Source: three-view drawing plus pictorial views. Frame: mm from the lowest corner of the part. A direction names the side the tool comes from. Coordinates: 2 decimals unless noted, no trailing zeros. Write each loop counter-clockwise with the first axis right and the second up, starting at its lowest first coordinate (ties: lowest second). Pieces come first, ordered by that corner, then holes. Notation, with made-up numbers: (70, 55) - (124, 55) arc R13 ccw to (124, 74) - close; hole circle Ø7 at (-34, 56). An arc over 180 degrees is marked (long way). Put each result on its own line as item: value.
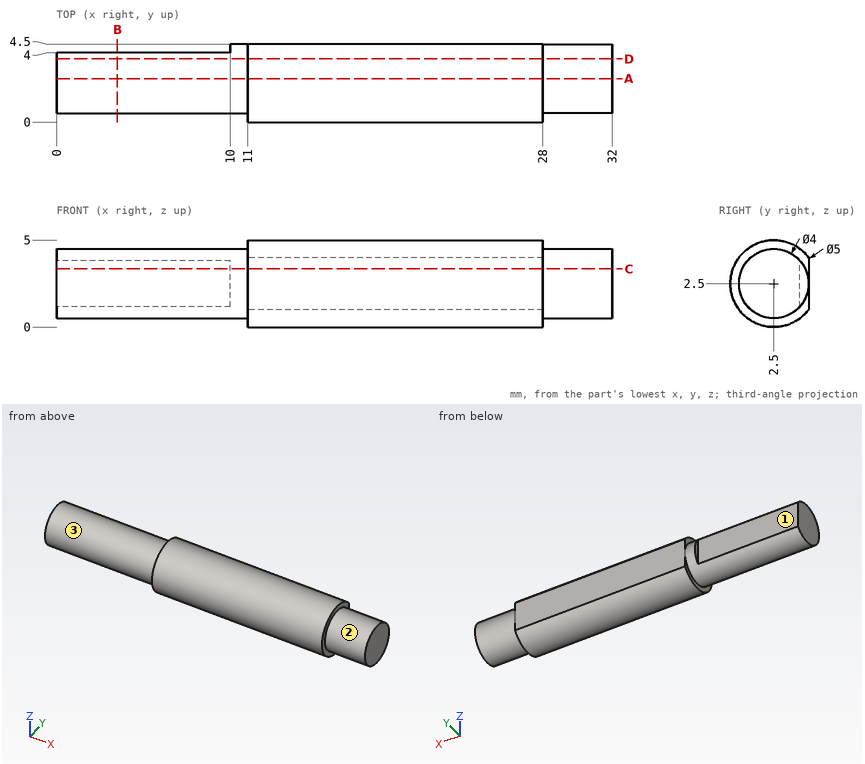
1. Section query B-B (x = 3.5). Return loops of the section in (y, z).
Answer below:
outline: (4, 1.18) - (4, 3.82) arc R2 ccw (long way) to start
2. Section query D-D (y = 3.65). Return loops of the section in (x, z), then the cut area to 3 significant figures.
Answer below:
outline: (0, 0.86) - (11, 0.86) - (11, 0.28) - (28, 0.28) - (28, 0.86) - (32, 0.86) - (32, 4.14) - (28, 4.14) - (28, 4.72) - (11, 4.72) - (11, 4.14) - (0, 4.14) - close
area: 125 mm²
3. Section query C-C (z = 3.35). Return loops of the section in (x, y), then the cut area to 3 significant figures.
Answer below:
outline: (0, 0.69) - (11, 0.69) - (11, 0.15) - (28, 0.15) - (28, 0.69) - (32, 0.69) - (32, 4.31) - (28, 4.31) - (28, 4.5) - (11, 4.5) - (11, 4.31) - (10, 4.31) - (10, 4) - (0, 4) - close
area: 125 mm²
4. Set-up query: the marked faces 1, 2 and 3. Return all of +Z, -Z, +X, -X, +Y, -Y with unobstructed straight access to the full face (end or side cutting, diameter ignored); none if empty.
Answer below:
face 1: +Z, -Z, -X, +Y
face 2: +X
face 3: -X
5. Ray query, probe 1 along Y at (x, z) = (7.5, 2.6); probe 2 along Y at (x, z) = (16, 2.35); probe 3 along X at (y, z) = (4.3, 1.4). Return the intervals inside material, ascending. Write a range as from..to.
Answer below:
probe 1: y = 0.5..4
probe 2: y = 0..4.5
probe 3: x = 11..28
6. Pin query (flat end, axial travel): pin 1 Ø0.8 at (x, z) = (5, 3) entering from +Y. Return the tip coordinate at first contact, or that it passes through.
Answer below:
pin 1: stops at y = 4
7. Section query A-A (y = 2.5). Return loops of the section in (x, z).
Answer below:
outline: (0, 0.5) - (11, 0.5) - (11, 0) - (28, 0) - (28, 0.5) - (32, 0.5) - (32, 4.5) - (28, 4.5) - (28, 5) - (11, 5) - (11, 4.5) - (0, 4.5) - close
